from build123d import *

# Parameters (mm, degrees)
EXTRUDE_1_DEPTH      = 1100
EXTRUDE_1_DEPTH_BACK = 90
SKETCH_1_W           = 22
SKETCH_1_H           = 22
SKETCH_2_W           = 22
SKETCH_2_H           = 22
EXTRUDE_2_DEPTH      = 130
SKETCH1_W            = 17
SKETCH1_H            = 17
CUT_EXTRUDE1_DEPTH   = 1321.091663484
FILLET2_R            = 6
FILLET3_R            = 4


with BuildPart() as part:
    # Эскиз1 → Бобышка-Вытянуть1 (new, two sides: drawn at the far end of the back side and taken through both)
    with BuildSketch(Plane(origin=(0, 0, 0), x_dir=(1, 0, 0), z_dir=(0, 1, 0)).offset(-EXTRUDE_1_DEPTH_BACK)):
        Rectangle(SKETCH_1_W, SKETCH_1_H)
    extrude(amount=EXTRUDE_1_DEPTH + EXTRUDE_1_DEPTH_BACK)

    # Эскиз2 → Бобышка-Вытянуть2 (add)
    with BuildSketch(Plane.XZ.offset(90)):
        Rectangle(SKETCH_2_W, SKETCH_2_H)
    extrude(amount=EXTRUDE_2_DEPTH)

    # Sketch1 → Cut-Extrude1 (cut, through all)
    with BuildSketch(Plane.XZ.offset(220)):
        Rectangle(SKETCH1_W, SKETCH1_H)
    extrude(amount=-CUT_EXTRUDE1_DEPTH, mode=Mode.SUBTRACT)

    # Fillet2
    fillet2_edges = [part.edges().sort_by_distance(p)[0] for p in [
        (11, 440, 11),
        (-11, 440, 11),
        (-11, 440, -11),
        (11, 440, -11),
    ]]
    fillet(fillet2_edges, radius=FILLET2_R)

    # Fillet3
    fillet3_edges = [part.edges().sort_by_distance(p)[0] for p in [
        (8.5, 440, 8.5),
        (8.5, 440, -8.5),
        (-8.5, 440, -8.5),
        (-8.5, 440, 8.5),
    ]]
    fillet(fillet3_edges, radius=FILLET3_R)


solid = part.part
Geometry check sheet. Reference: the model listing, model coordinates, mm. Round coordinates to 2 decimals unless told otherwise and drop trailing zeros. Write each loop counter-clockwise with the first axis right and the second up, starting at its lowest first coordinate (ties: lowest second). Pieces come first, ordered by that corner, then holes. Notation, with made-up numbers: (-32, 56.25) -> (9, 56.25) arc R9 ccw to (9, 66.25) -> close; hole circle Ø10 at (70.5, 9.25). An arc over 180 degrees is marked (long way). One line per item, written item: value. Start each with the question number.
(1) Go/stop test with a flat-tipped pin: pin 1 Ø10 at (y, z) = (578, 8.5) entering from +X. Record where the tip stops, or that it passes through.
(2) Cross-section at B-B, the plane y = 725. Record the cut outline in (x, z).
(3) Cross-section at A-A, the plane x = 0.75. Record the cut outline in (y, z).
(4) Scan lines: line 1 (X direction, y = 235, z = 2.75); line 2 (Z direction, x = -5.5, y = 237). Record each from-to range of solid material in increasing order. Write a range as [from, to].
Answer:
1. pin 1: x = 11
2. outline: (-11, -5) arc R6 ccw to (-5, -11) -> (5, -11) arc R6 ccw to (11, -5) -> (11, 5) arc R6 ccw to (5, 11) -> (-5, 11) arc R6 ccw to (-11, 5) -> close; hole (-8.5, -4.5) arc R4 ccw to (-4.5, -8.5) -> (4.5, -8.5) arc R4 ccw to (8.5, -4.5) -> (8.5, 4.5) arc R4 ccw to (4.5, 8.5) -> (-4.5, 8.5) arc R4 ccw to (-8.5, 4.5) -> close
3. outline: (-220, -11) -> (1100, -11) -> (1100, -8.5) -> (-220, -8.5) -> close; (-220, 8.5) -> (1100, 8.5) -> (1100, 11) -> (-220, 11) -> close
4. line 1: [-11, -8.5], [8.5, 11]
4. line 2: [-10.98, -8.37], [8.37, 10.98]
